The model under review builds one solid part; all positions refer to its coordinate system, in mm. A direction names the side the tool comes from. Round coordinates to 2 decimals unless told otherwise and drop trailing zeros. Write each loop counter-clockwise with the first axis right and the second up, starting at its lowest first coordinate (ties: lowest second). Pieces come first, ordered by that corner, then holes. Notation, with made-up numbers: (-5.5, 44.5) - (41.5, 44.5) arc R6 ccw to (41.5, 53.5) - close; hole circle Ø8 at (17, 48). An arc over 180 degrees is marked (long way). One line per question, with ' | ' between items. Start each with the question number.
```python
from build123d import *


with BuildPart() as part:
    # Esquisse1 → Révolution1 (revolve)
    with BuildSketch(Plane.XY):
        with BuildLine():
            Line((0, 4.3), (-27.5, 4.3))
            ThreePointArc((-27.5, 4.3), (-28.065685425, 4.065685425), (-28.3, 3.5))
            Line((-28.3, 3.5), (-28.3, 3.35))
            Line((-28.3, 3.35), (-29.25, 3.35))
            Line((-29.25, 3.35), (-29.25, 4.45))
            ThreePointArc((-29.25, 4.45), (-29.015685425, 5.015685425), (-28.45, 5.25))
            Line((-28.45, 5.25), (-0.95, 5.25))
            Line((-0.95, 5.25), (-0.95, 5.9))
            Line((-0.95, 5.9), (0, 5.9))
            Line((0, 5.9), (0, 5.25))
            Line((0, 5.25), (0, 4.3))
        make_face()
    revolve(axis=Axis((0, 0, 0), (-1, 0, 0)))


solid = part.part
```
1. Machinability: for faces 1 (the face through (-13.942, -4.296, -0.189)), 2 (the face through (-14.5, 5, -1.6)), 3 (the face through (-29.25, 2, -3)), which of the approach directions +Z, -Z, +X, -X, +Y, -Y give a long, thin tool a straight path to every point of the face, cutting with its end or side? Answer none if there is none.
2. Clearance check with flat-ended pins moving along their axes: P1, Ø5.5, axis at y = 0, z = 0, coming from the +X side; P2, Ø5, axis at x = -12.5, y = 2.5, coming from the +Z side; P3, Ø3, axis at x = -19, z = -1, coming from the -Y side; P4, Ø5.5, axis at y = 1.5, z = -1.5, coming from the +X side. State where each tip first meets the part, or that it passes through.
3. Add section C-C, the plane x = -24.75. Write out the cut boundary in (y, z).
4. Add section A-A, the plane y = 0. Write out the cut boundary in (x, z), then the cut area to 3 significant figures.
5. The part is to be moulded in two halves that separate along Z. For faces 4 (the face through (0, -4, 2)), 5 (the face through (-0.468, -5.894, -0.259)), 6 (the face through (-28.782, -3.347, -0.147)), say which applies: pulls with the +Z half, pulls with the -Z half, needs draft (parallel to the pull), parting line crosses it, or undercut.
6. Wall thickness on line 1 along Z through (x, y) = (-17.25, 0); line 2 along X through (y, z) = (-2.75, -2); line 3 along X through (y, z) = (1.75, 5): over which ranges is each line inside the solid? List them lowest first. Write a range as [from, to].
Geometry check:
1) face 1: +X | face 2: -X | face 3: +Z, -Z, -X, +Y, -Y
2) P1: passes through | P2: stops at z = 5.25 | P3: stops at y = -5.25 | P4: stops at x = 0
3) outline: circle Ø10.5 at (0, 0); hole circle Ø8.6 at (0, 0)
4) outline: (-29.25, -4.45) arc R0.8 ccw to (-28.45, -5.25) - (-0.95, -5.25) - (-0.95, -5.9) - (0, -5.9) - (0, -4.3) - (-27.5, -4.3) arc R0.8 cw to (-28.3, -3.5) - (-28.3, -3.35) - (-29.25, -3.35) - close; (-29.25, 3.35) - (-28.3, 3.35) - (-28.3, 3.5) arc R0.8 cw to (-27.5, 4.3) - (0, 4.3) - (0, 5.9) - (-0.95, 5.9) - (-0.95, 5.25) - (-28.45, 5.25) arc R0.8 ccw to (-29.25, 4.45) - close | area: 58.6 mm2
5) face 4: needs draft | face 5: parting line crosses it | face 6: undercut
6) line 1: z = [-5.25, -4.3], [4.3, 5.25] | line 2: x = [-29.25, -28.3] | line 3: x = [-0.95, 0]
